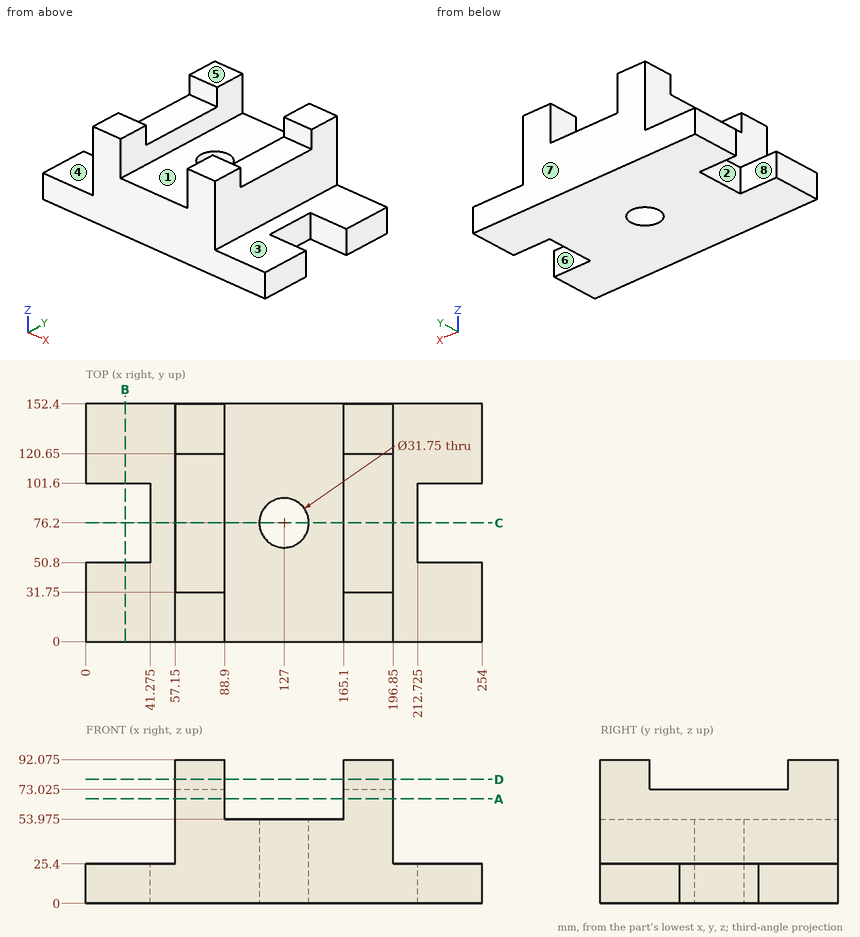
Can you work these out from the drawing? Everything is in mm from the part's minimum corner. A direction names the side the tool comes from. Give positions to 0.01 mm unless a question says otherwise; leave off trailing zeros. Loops run counter-clockwise (first coordinate to the right, second up) from the corner with the lowest first, then second, coordinate; pieces in that order, holes last. Notation, with made-up numbers: (71.5, -21) - (99.5, -21) arc R23 cw to (99.5, 12) - close; hole circle Ø3 at (-13, 24). An arc over 180 degrees is marked (long way). Answer as a JSON object with one key per item and string values.
Q1. Imagine slicing it at B-B on x = 25. Write out the boundary of the cut face in (y, z), plus the area to 3 significant figures.
Geometry says:
{"outline": "(0, 0) - (50.8, 0) - (50.8, 25.4) - (0, 25.4) - close; (101.6, 0) - (152.4, 0) - (152.4, 25.4) - (101.6, 25.4) - close", "area": "2,580 mm²"}
Q2. Will these pins go through, and if not, where does the flat tip stop? P1, Ø12, axis at y = 135.5, z = 33, coming from the +X side; P2, Ø17, axis at x = 42, y = 50.5, coming from the +Z side; P3, Ø12, axis at y = 104, z = 39, coming from the -X side.
Geometry says:
{"P1": "x = 196.85", "P2": "z = 25.4", "P3": "x = 57.15"}
Q3. Which directions (+Z, -Z, +X, -X, +Y, -Y) give clear straight access to the entire face, cutting with the end or side of a thin tool? Please do the marked faces 1, 2, 3 and 4.
Geometry says:
{"face 1": "+Z, +Y, -Y", "face 2": "+Z, -Z, -X", "face 3": "+Z, +X, +Y, -Y", "face 4": "+Z, -X, +Y, -Y"}
Q4. Imagine slicing it at D-D on z = 79.5. Write out the boundary of the cut face in (x, y), plus the area to 3 significant figures.
Geometry says:
{"outline": "(57.15, 0) - (88.9, 0) - (88.9, 31.75) - (57.15, 31.75) - close; (57.15, 120.65) - (88.9, 120.65) - (88.9, 152.4) - (57.15, 152.4) - close; (165.1, 0) - (196.85, 0) - (196.85, 31.75) - (165.1, 31.75) - close; (165.1, 120.65) - (196.85, 120.65) - (196.85, 152.4) - (165.1, 152.4) - close", "area": "4,030 mm²"}
Q5. If we mould it in two halves opening along Y, with no side actions, what happens to the marked faces 5, 6, 7 and 8? For each: pulls with the +Y half, pulls with the -Y half, needs draft (parallel to the pull), parting line crosses it, or undercut.
Geometry says:
{"face 5": "needs draft", "face 6": "undercut", "face 7": "pulls with the +Y half", "face 8": "undercut"}
Q6. Imagine slicing it at A-A on z = 67. Write out the boundary of the cut face in (x, y).
Geometry says:
{"outline": "(57.15, 0) - (88.9, 0) - (88.9, 152.4) - (57.15, 152.4) - close; (165.1, 0) - (196.85, 0) - (196.85, 152.4) - (165.1, 152.4) - close"}
Q7. If I drill on L1, parallel to X at y = 118, z = 68; L2, parallel to X at y = 76, z = 38; L3, parallel to Y at x = 127, z = 30.5 (3 decimals), over which ranges is the centre line in solid material (lowest first)?
Geometry says:
{"L1": "57.15 to 88.9, 165.1 to 196.85", "L2": "57.15 to 111.13, 142.87 to 196.85", "L3": "0 to 60.325, 92.075 to 152.4"}
Q8. Imagine slicing it at C-C on y = 76.2. Write out the boundary of the cut face in (x, z) (3 decimals).
Geometry says:
{"outline": "(41.275, 0) - (111.125, 0) - (111.125, 53.975) - (88.9, 53.975) - (88.9, 73.025) - (57.15, 73.025) - (57.15, 25.4) - (41.275, 25.4) - close; (142.875, 0) - (212.725, 0) - (212.725, 25.4) - (196.85, 25.4) - (196.85, 73.025) - (165.1, 73.025) - (165.1, 53.975) - (142.875, 53.975) - close"}
